from build123d import *

# Parameters (mm, degrees)
SKETCH_1_R          = 6
EXTRUDE_1_DEPTH     = 2
FILLET_1_R          = 1
SKETCH_2_R          = 1.515
CUT_EXTRUDE_1_DEPTH = 10
CUT_EXTRUDE_2_DEPTH = 10
FILLET_2_R          = 1.3


with BuildPart() as part:
    # 草图1 → 凸台-拉伸1 (new body)
    with BuildSketch(Plane.XY):
        with BuildLine():
            Line((-20, -25), (20, -25))
            Line((20, -25), (20, -19))
            Line((20, -19), (11.781235871, 4.177616707))
            ThreePointArc((11.781235871, 4.177616707), (0, 12.5), (-11.781235871, 4.177616707))
            Line((-11.781235871, 4.177616707), (-20, -19))
            Line((-20, -19), (-20, -25))
        make_face()
        Circle(SKETCH_1_R, mode=Mode.SUBTRACT)
    extrude(amount=EXTRUDE_1_DEPTH)

    # 圆角1
    fillet_1_edges = [part.edges().sort_by_distance(p)[0] for p in [
        (20, -19, 1),
        (20, -25, 1),
        (-20, -25, 1),
        (-20, -19, 1),
    ]]
    fillet(fillet_1_edges, radius=FILLET_1_R)

    # 草图2 → 切除-拉伸1 (cut)
    with BuildSketch(Plane(origin=(0, 0, 0), x_dir=(-1, 0, 0), z_dir=(0, 0, -1))):
        with Locations((15, -22)):
            Circle(SKETCH_2_R)
        with Locations((-5, -22)):
            Circle(SKETCH_2_R)
    extrude(amount=-CUT_EXTRUDE_1_DEPTH, mode=Mode.SUBTRACT)

    # 草图3 → 切除-拉伸2 (cut)
    with BuildSketch(Plane(origin=(0, 0, 0), x_dir=(-1, 0, 0), z_dir=(0, 0, -1))):
        with BuildLine():
            Line((-9.252304266, -2.155195065), (-15.225458465, -19))
            Line((-15.225458465, -19), (15.225458465, -19))
            Line((15.225458465, -19), (9.252304266, -2.155195065))
            ThreePointArc((9.252304266, -2.155195065), (0, -9.5), (-9.252304266, -2.155195065))
        make_face()
    extrude(amount=-CUT_EXTRUDE_2_DEPTH, mode=Mode.SUBTRACT)

    # 圆角2
    fillet_2_edges = [part.edges().sort_by_distance(p)[0] for p in [
        (9.252304266, -2.155195065, 1),
        (-9.252304266, -2.155195065, 1),
        (-15.225458465, -19, 1),
        (15.225458465, -19, 1),
    ]]
    fillet(fillet_2_edges, radius=FILLET_2_R)


solid = part.part
The model under review builds one solid part; all positions refer to its coordinate system, in mm. A direction names the side the tool comes from. Round coordinates to 2 decimals unless told otherwise and drop trailing zeros. Write each loop counter-clockwise with the first axis right and the second up, starting at its lowest first coordinate (ties: lowest second). Pieces come first, ordered by that corner, then holes. Notation, with made-up numbers: M 35.5,-28.5 L 69.5,-28.5 A25 ccw 69.5,-3.5 Z; hole C -32.75,56.25 d2. An arc over 180 degrees is marked long. Use a Markdown table: item, result. Add a question column.
Q1. Insertion check: pin 1 (5 mm diameter, centred on x = 5, y = -22, fed in from -Z). The pin has a flat end and moves straight along its axis. Give the tip position at first contact, or say it passes through.
Q2. The part is to be moulded in two halves that separate along X. For faces 3 (the face through (19.699, -24.715, 1.014)), 4 (the face through (12.46, -11.2, 0.99)), 5 (the face through (-20, -22, 1)), 6 (the face through (4.301, -23.344, 0.986)), say which applies: pulls with the +X half, pulls with the -X half, needs draft (parallel to the pull), parting line crosses it, or undercut.
Q3. We need section B-B, the plane x = 0. State the section outline as (y, z) points, plus the area to 3 significant figures.
Q4. Machinability: for faces 1 (the face through (-12.52, -11.37, 0.99)), 2 (the face through (0, -25, 1)), which of the approach directions +Z, -Z, +X, -X, +Y, -Y give a long, thin tool a straight path to every point of the face, cutting with its end or side? Answer none if there is none.
Q5. We need section A-A, the plane y = -22. State the section outline as (x, z) points (3 decimals).
Q6. We need section D-D, the plane y = -13.5. State the section outline as (x, z) points.
Q7. We need section C-C, the plane z = 0.65. Count the separate pieces of the cut face and the enclosed holes in it, plus the area to 3 significant figures.
Q8. To check wall thickness, follow line 1 (Y direction, x = 0, z = 0.55); line 2 (X direction, y = -7.5, z = 0.75); line 3 (X direction, y = -8, z = 0.9). State the ranges of each line that lie inside material, in increasing order.
Findings below:
| question | item | result |
|---|---|---|
| 1 | pin 1 | stops at z = 0 |
| 2 | face 3 | pulls with the +X half |
| 2 | face 4 | undercut |
| 2 | face 5 | pulls with the -X half |
| 2 | face 6 | undercut |
| 3 | outline | M -25,0 L -19,0 L -19,2 L -25,2 Z; M -9.5,0 L -6,0 L -6,2 L -9.5,2 Z; M 6,0 L 12.5,0 L 12.5,2 L 6,2 Z |
| 3 | area | 32.0 mm² |
| 4 | face 1 | +Z, -Z |
| 4 | face 2 | +Z, -Z, +X, -X, -Y |
| 5 | outline | M -20,0 L -16.515,0 L -16.515,2 L -20,2 Z; M -13.485,0 L 3.485,0 L 3.485,2 L -13.485,2 Z; M 6.515,0 L 20,0 L 20,2 L 6.515,2 Z |
| 6 | outline | M -18.05,0 L -13.28,0 L -13.28,2 L -18.05,2 Z; M 13.28,0 L 18.05,0 L 18.05,2 L 13.28,2 Z |
| 7 | separate pieces | 1 |
| 7 | enclosed holes | 4 |
| 7 | area | 686 mm² |
| 8 | line 1 | y = -25 to -19, -9.5 to -6, 6 to 12.5 |
| 8 | line 2 | x = -15.92 to -11.15, -5.83 to 5.83, 11.15 to 15.92 |
| 8 | line 3 | x = -16.1 to -11.32, -5.12 to 5.12, 11.32 to 16.1 |
